Could you check a few things on this model? Use its own coordinates, in mm. A direction names the side the tool comes from. Give positions to 0.01 mm unless a question says otherwise; leave off trailing zeros. Loops run counter-clockwise (first coordinate to the right, second up) from the corner with the lowest first, then second, coordinate; pieces in that order, holes last. Notation, with made-up numbers: (2.5, 23.5) -> (53.5, 23.5) arc R17 cw to (53.5, 33.5) -> close; hole circle Ø6 at (-32.75, 60). An arc over 180 degrees is marked (long way). Put each result on its own line as item: value.
```python
from build123d import *

# Parameters (mm, degrees)
PAD018_DEPTH           = 12
CYLINDER023_R          = 4.5
CYLINDER023_DEPTH      = 12
PAD019_DEPTH           = 5
CUT017_PLACEMENT_ANGLE = 180


with BuildPart() as body016:
    # Sketch153 → Pad018 (new body)
    with BuildSketch(Plane.XY):
        with BuildLine():
            ThreePointArc((-1.924981, -2.651228), (3.274094, -0.001028), (-1.924981, 2.649172))
            Line((-1.924981, 2.649172), (-1.924981, -2.651228))
        make_face()
    extrude(amount=PAD018_DEPTH)


with BuildPart() as cylinder023:
    # Cylinder023 → Cylinder023 (new body)
    with BuildSketch(Plane.XY):
        Circle(CYLINDER023_R)
    extrude(amount=CYLINDER023_DEPTH)


with BuildPart() as pinion001:
    # Sketch154 → Pad019 (new body)
    with BuildSketch(Plane.XY):
        with BuildLine():
            Line((5.562447, 1.006802), (5.903793, 1.165811))
            Line((5.903793, 1.165811), (6.726635, 1.937659))
            ThreePointArc((6.726635, 1.937659), (6.634334, 2.233423), (6.529036, 2.524814))
            Line((6.529036, 2.524814), (5.406959, 2.642124))
            Line((5.406959, 2.642124), (5.03893, 2.562402))
            Line((5.03893, 2.562402), (4.554688, 2.317075))
            ThreePointArc((4.06426, 2.456563), (4.282119, 2.290644), (4.554688, 2.317075))
            ThreePointArc((4.06426, 2.456563), (3.955033, 2.628881), (3.838507, 2.796349))
            ThreePointArc((3.899966, 3.30251), (3.769976, 3.061482), (3.838507, 2.796349))
            Line((3.899966, 3.30251), (4.313775, 3.653848))
            Line((4.313775, 3.653848), (4.529885, 3.962227))
            Line((4.529885, 3.962227), (4.856563, 5.042087))
            ThreePointArc((4.856563, 5.042087), (4.628746, 5.252076), (4.39186, 5.451779))
            Line((4.39186, 5.451779), (3.361458, 4.992334))
            Line((3.361458, 4.992334), (3.082596, 4.739278))
            Line((3.082596, 4.739278), (2.785893, 4.284698))
            ThreePointArc((2.291426, 4.160284), (2.563058, 4.125524), (2.785893, 4.284698))
            ThreePointArc((2.291426, 4.160284), (2.110674, 4.254902), (1.926025, 4.34167))
            ThreePointArc((1.72617, 4.810749), (1.734109, 4.537017), (1.926025, 4.34167))
            Line((1.72617, 4.810749), (1.90887, 5.321921))
            Line((1.90887, 5.321921), (1.941838, 5.697039))
            Line((1.941838, 5.697039), (1.684819, 6.795565))
            ThreePointArc((1.684819, 6.795565), (1.382529, 6.863512), (1.077528, 6.918017))
            Line((1.077528, 6.918017), (0.414896, 6.004925))
            Line((0.414896, 6.004925), (0.299923, 5.646341))
            Line((0.299923, 5.646341), (0.270261, 5.104312))
            ThreePointArc((-0.095753, 4.749333), (0.156867, 4.855045), (0.270261, 5.104312))
            ThreePointArc((-0.095753, 4.749333), (-0.299598, 4.740898), (-0.502893, 4.723717))
            ThreePointArc((-0.910512, 5.030024), (-0.76677, 4.796935), (-0.502893, 4.723717))
            Line((-0.910512, 5.030024), (-1.007875, 5.564062))
            Line((-1.007875, 5.564062), (-1.166883, 5.905408))
            Line((-1.166883, 5.905408), (-1.938731, 6.72825))
            ThreePointArc((-1.938731, 6.72825), (-2.234496, 6.635949), (-2.525886, 6.53065))
            Line((-2.525886, 6.53065), (-2.643196, 5.408573))
            Line((-2.643196, 5.408573), (-2.563474, 5.040545))
            Line((-2.563474, 5.040545), (-2.318147, 4.556302))
            ThreePointArc((-2.457636, 4.065874), (-2.291717, 4.283734), (-2.318147, 4.556302))
            ThreePointArc((-2.457636, 4.065874), (-2.629953, 3.956647), (-2.797421, 3.840121))
            ThreePointArc((-3.303583, 3.90158), (-3.062555, 3.77159), (-2.797421, 3.840121))
            Line((-3.303583, 3.90158), (-3.65492, 4.315389))
            Line((-3.65492, 4.315389), (-3.963299, 4.531499))
            Line((-3.963299, 4.531499), (-5.04316, 4.858177))
            ThreePointArc((-5.04316, 4.858177), (-5.253149, 4.63036), (-5.452851, 4.393474))
            Line((-5.452851, 4.393474), (-4.993407, 3.363072))
            Line((-4.993407, 3.363072), (-4.740351, 3.084211))
            Line((-4.740351, 3.084211), (-4.28577, 2.787507))
            ThreePointArc((-4.161356, 2.29304), (-4.126596, 2.564672), (-4.28577, 2.787507))
            ThreePointArc((-4.161356, 2.29304), (-4.255974, 2.112288), (-4.342743, 1.927639))
            ThreePointArc((-4.811821, 1.727784), (-4.53809, 1.735724), (-4.342743, 1.927639))
            Line((-4.811821, 1.727784), (-5.322993, 1.910485))
            Line((-5.322993, 1.910485), (-5.698112, 1.943452))
            Line((-5.698112, 1.943452), (-6.796638, 1.686433))
            ThreePointArc((-6.796638, 1.686433), (-6.864585, 1.384143), (-6.919089, 1.079142))
            Line((-6.919089, 1.079142), (-6.005997, 0.41651))
            Line((-6.005997, 0.41651), (-5.647414, 0.301537))
            Line((-5.647414, 0.301537), (-5.105384, 0.271875))
            ThreePointArc((-4.750405, -0.094139), (-4.856118, 0.158481), (-5.105384, 0.271875))
            ThreePointArc((-4.750405, -0.094139), (-4.74197, -0.297984), (-4.72479, -0.501279))
            ThreePointArc((-5.031096, -0.908898), (-4.798007, -0.765156), (-4.72479, -0.501279))
            Line((-5.031096, -0.908898), (-5.565134, -1.00626))
            Line((-5.565134, -1.00626), (-5.90648, -1.165269))
            Line((-5.90648, -1.165269), (-6.729322, -1.937117))
            ThreePointArc((-6.729322, -1.937117), (-6.637021, -2.232881), (-6.531723, -2.524272))
            Line((-6.531723, -2.524272), (-5.409646, -2.641582))
            Line((-5.409646, -2.641582), (-5.041617, -2.56186))
            Line((-5.041617, -2.56186), (-4.557374, -2.316533))
            ThreePointArc((-4.066946, -2.456021), (-4.284806, -2.290102), (-4.557374, -2.316533))
            ThreePointArc((-4.066946, -2.456021), (-3.957719, -2.628339), (-3.841193, -2.795807))
            ThreePointArc((-3.902653, -3.301969), (-3.772663, -3.06094), (-3.841193, -2.795807))
            Line((-3.902653, -3.301969), (-4.316462, -3.653306))
            Line((-4.316462, -3.653306), (-4.532572, -3.961685))
            Line((-4.532572, -3.961685), (-4.85925, -5.041545))
            ThreePointArc((-4.85925, -5.041545), (-4.631433, -5.251535), (-4.394546, -5.451237))
            Line((-4.394546, -5.451237), (-3.364144, -4.991792))
            Line((-3.364144, -4.991792), (-3.085283, -4.738736))
            Line((-3.085283, -4.738736), (-2.78858, -4.284156))
            ThreePointArc((-2.294113, -4.159742), (-2.565744, -4.124982), (-2.78858, -4.284156))
            ThreePointArc((-2.294113, -4.159742), (-2.11336, -4.25436), (-1.928712, -4.341129))
            ThreePointArc((-1.728857, -4.810207), (-1.736796, -4.536475), (-1.928712, -4.341129))
            Line((-1.728857, -4.810207), (-1.911557, -5.321379))
            Line((-1.911557, -5.321379), (-1.944525, -5.696498))
            Line((-1.944525, -5.696498), (-1.687506, -6.795023))
            ThreePointArc((-1.687506, -6.795023), (-1.385216, -6.862971), (-1.080215, -6.917475))
            Line((-1.080215, -6.917475), (-0.417583, -6.004383))
            Line((-0.417583, -6.004383), (-0.30261, -5.6458))
            Line((-0.30261, -5.6458), (-0.272948, -5.10377))
            ThreePointArc((0.093067, -4.748791), (-0.159553, -4.854503), (-0.272948, -5.10377))
            ThreePointArc((0.093067, -4.748791), (0.296912, -4.740356), (0.500206, -4.723176))
            ThreePointArc((0.907825, -5.029482), (0.764084, -4.796393), (0.500206, -4.723176))
            Line((0.907825, -5.029482), (1.005188, -5.56352))
            Line((1.005188, -5.56352), (1.164197, -5.904866))
            Line((1.164197, -5.904866), (1.936044, -6.727708))
            ThreePointArc((1.936044, -6.727708), (2.231809, -6.635407), (2.523199, -6.530108))
            Line((2.523199, -6.530108), (2.64051, -5.408032))
            Line((2.64051, -5.408032), (2.560787, -5.040003))
            Line((2.560787, -5.040003), (2.315461, -4.55576))
            ThreePointArc((2.454949, -4.065332), (2.28903, -4.283192), (2.315461, -4.55576))
            ThreePointArc((2.454949, -4.065332), (2.627267, -3.956105), (2.794735, -3.839579))
            ThreePointArc((3.300896, -3.901038), (3.059868, -3.771048), (2.794735, -3.839579))
            Line((3.300896, -3.901038), (3.652234, -4.314848))
            Line((3.652234, -4.314848), (3.960612, -4.530958))
            Line((3.960612, -4.530958), (5.040473, -4.857636))
            ThreePointArc((5.040473, -4.857636), (5.250462, -4.629818), (5.450164, -4.392932))
            Line((5.450164, -4.392932), (4.99072, -3.36253))
            Line((4.99072, -3.36253), (4.737664, -3.083669))
            Line((4.737664, -3.083669), (4.283083, -2.786966))
            ThreePointArc((4.15867, -2.292498), (4.123909, -2.56413), (4.283083, -2.786966))
            ThreePointArc((4.15867, -2.292498), (4.253288, -2.111746), (4.340056, -1.927098))
            ThreePointArc((4.809135, -1.727242), (4.535403, -1.735182), (4.340056, -1.927098))
            Line((4.809135, -1.727242), (5.320306, -1.909943))
            Line((5.320306, -1.909943), (5.695425, -1.94291))
            Line((5.695425, -1.94291), (6.793951, -1.685891))
            ThreePointArc((6.793951, -1.685891), (6.861898, -1.383601), (6.916402, -1.078601))
            Line((6.916402, -1.078601), (6.003311, -0.415969))
            Line((6.003311, -0.415969), (5.644727, -0.300996))
            Line((5.644727, -0.300996), (5.102697, -0.271334))
            ThreePointArc((4.747718, 0.094681), (4.853431, -0.157939), (5.102697, -0.271334))
            ThreePointArc((4.747718, 0.094681), (4.739284, 0.298526), (4.722103, 0.501821))
            ThreePointArc((5.028409, 0.909439), (4.795321, 0.765698), (4.722103, 0.501821))
            Line((5.028409, 0.909439), (5.562447, 1.006802))
        make_face()
    extrude(amount=PAD019_DEPTH)

    # Fusion024: union Cylinder023
    add(cylinder023.part)

    # Cut017: cut Body016
    add(body016.part, mode=Mode.SUBTRACT)


with BuildPart() as pinion001_1:
    # Cut017 placement: moved
    add(pinion001.part.moved(Location((43.9, 2.76, 35))).rotate(Axis((43.9, 2.76, 35), (1, 0, 0)), CUT017_PLACEMENT_ANGLE))


solid = pinion001_1.part
```
1. I'm going to push flat-ended pins straight in: pin 1 (6 mm diameter, centred on x = 49, z = 32, fed in from -Y); pin 2 (1.6 mm diameter, centred on y = 1.5, z = 30, fed in from +X); pin 3 (5 mm diameter, centred on y = -2, z = 33.5, fed in from -X). Where does each tip first touch, or does it pass through?
Recorded:
pin 1: stops at y = -2.69
pin 2: stops at x = 50.63
pin 3: stops at x = 38.45
2. If we section it at A-A (z = 28): List the corners of the cut face in (x, y) for me (3 decimals), then the cut area to 3 significant figures.
Recorded:
outline: circle Ø9 at (43.9, 2.76); hole (41.975, 0.111) arc R3.275 ccw (long way) to (41.975, 5.411) -> close
area: 34.9 mm^2
3. I need wall thicknesses on line 1 (Y direction, x = 46.25, z = 28.25); line 2 (X direction, y = 2.75, z = 26); line 3 (X direction, y = -2.5, z = 32.5). Which ranges of each line are inside material? Lowest first, please.
Recorded:
line 1: y = -1.08 to 0.48, 5.04 to 6.6
line 2: x = 39.4 to 41.98, 47.17 to 48.4
line 3: x = 41.29 to 42.95, 44.18 to 45.79, 47.86 to 48.52
4. For faces 1 (the face through (41.975, 3, 29)), 2 (the face through (50.209, 1.214, 32.535)), 3 (the face through (37.431, 2.008, 32.535)), 4 (the face through (39.404, -1.933, 32.535)), which set-ups out of +Z, -Z, +X, -X, +Y, -Y let a thin tool reach every point of the face, with its end or its side?
Recorded:
face 1: +Z, -Z
face 2: +Z, -Z, +X
face 3: +Z, -Z, -X
face 4: +Z, -Z, -Y
5. Thinking about a two-plate mould opening in X: for faces 5 (the face through (50.137, 4.576, 32.535)), 6 (the face through (42.92, 7.15, 26.55)), 7 (the face through (40.013, 7.985, 32.535)), 8 (the face through (44.65, -3.71, 32.54)), which applies, pulls with the +X half, pulls with the -X half, needs draft (parallel to the pull), parting line crosses it, or undercut?
Recorded:
face 5: pulls with the +X half
face 6: parting line crosses it
face 7: undercut
face 8: undercut
